Verification items for the finished model (mm, model axes). A direction names the side the tool comes from. Round coordinates to 2 decimals unless told otherwise and drop trailing zeros. Loops run counter-clockwise (first coordinate to the right, second up) from the corner with the lowest first, then second, coordinate; pieces in that order, holes last. Notation, with made-up numbers: M 17.5,-25 L 22.5,-25 A15 cw 22.5,4 Z; hole C 47.5,84.25 d7. An arc over 180 degrees is marked long. One line per item, written item: value.
from build123d import *

# Parameters (mm, degrees)
CORTAR_EXTRUIR1_START = 9.5
CORTAR_EXTRUIR1_DEPTH = 7
CHAFL_N1_SIZE         = 0.8


with BuildPart() as part:
    # Croquis2 → Revolución1 (revolve)
    with BuildSketch(Plane.XY):
        Polygon((0, 0), (-12.5, 0), (-12.5, 10), (-8.5, 10), (-8.5, 15), (-12.5, 15), (-12.5, 178.3), (0, 200), align=None)
    revolve(axis=Axis((0, 200, 0), (0, -1, 0)))

    # Croquis3 → Cortar-Extruir1 (cut)
    with BuildSketch(Plane.XY.offset(CORTAR_EXTRUIR1_START)):
        with BuildLine():
            Line((3, 166.7), (3, 26.7))
            ThreePointArc((3, 26.7), (0, 23.7), (-3, 26.7))
            Line((-3, 26.7), (-3, 166.7))
            ThreePointArc((-3, 166.7), (0, 169.7), (3, 166.7))
        make_face()
    extrude(amount=CORTAR_EXTRUIR1_DEPTH, mode=Mode.SUBTRACT)

    # Chaflán1
    chafl_n1_edges = [part.edges().sort_by_distance(p)[0] for p in [
        (12.5, 15, 0),
        (12.5, 10, 0),
        (12.5, 0, 0),
    ]]
    chamfer(chafl_n1_edges, length=CHAFL_N1_SIZE)


solid = part.part
(1) Depth check by flat-ended pin: pin 1 Ø1.3 at (y, z) = (103, 11) entering from -X; pin 2 Ø1 at (y, z) = (26, -5) entering from +X; pin 3 Ø3 at (x, y) = (-2.5, 152.5) entering from -Z. Enter the tip coordinate at first touch or a pass-through.
Completed:
pin 1: stops at x = -7.01
pin 2: stops at x = 11.66
pin 3: stops at z = -12.46
(2) Sectioned sample at A-A on y = 93. Enter the section's corners in (x, z).
Completed:
outline: M -3,9.5 L -3,12.13 A12.5 ccw long 3,12.13 L 3,9.5 Z
(3) Tool access check on faces 5 (the face through (-8, 10, -4)), 6 (the face through (0, 98, 9.5)), 7 (the face through (-6.72, 98.19, -10.54)). Record the directions out of +Z, -Z, +X, -X, +Y, -Y that give a thin tool (end or side, any length) a straight path to the whole face; none if there is none.
Completed:
face 5: none
face 6: +Z
face 7: +Y, -Y
(4) Thickness scan on L1, parallel to Y at x = 9.75, z = -6; L2, parallel to Y at x = 2, z = -9.25; L3, parallel to Z at x = -4.5, y = 70. Record the ranges inside material, lowest first. Write a range as from..to.
Completed:
L1: y = 0..10, 15..180.13
L2: y = 0..10, 15..183.57
L3: z = -11.66..11.66
(5) Mould release check, pull along Y, two halves, no side actions. Record for faces 1 (the face through (0, 0, 0)), 2 (the face through (8, 15, -4)), 3 (the face through (-4.57, 12.535, -7.167)), 4 (the face through (-11.923, 5.059, -3.755)): +Y half, -Y half, draft (parallel to the pull), parting line (faces both ways), or undercut.
Completed:
face 1: -Y half
face 2: undercut
face 3: undercut
face 4: draft
